Can you work these out from the model? Positions are in its coordinate system, mm. Face numbers are marked on the shaded views. A direction names the side the tool comes from. Coordinates: 2 decimals unless noted, no trailing zeros. Write each loop counter-clockwise with the first axis right and the second up, starting at its lowest first coordinate (ties: lowest second). Pieces come first, ordered by that corner, then holes. Notation, with made-up numbers: M 84.25,28 L 125.25,28 A17 ccw 125.25,46 Z; hole C -39,-28 d11. An arc over 180 degrees is marked long. Use one line per item in the form item = value. Start each with the question number.
```python
from build123d import *

# Parameters (mm, degrees)
SKETCH_1_W          = 32.677388302
SKETCH_1_H          = 8
EXTRUDE_1_DEPTH     = 3
SKETCH_2_R          = 1.5
CUT_EXTRUDE_1_DEPTH = 4
SKETCH_3_R          = 6
EXTRUDE_2_DEPTH     = 8
SKETCH_4_R          = 4
CUT_EXTRUDE_2_DEPTH = 9
EXTRUDE_3_DEPTH     = 8
SKETCH_6_W          = 6
SKETCH_6_H          = 6
EXTRUDE_4_DEPTH     = 8
SKETCH_8_W          = 3
SKETCH_8_H          = 10.466633743
CUT_EXTRUDE_5_DEPTH = 9
SKETCH_9_R          = 1.5
CUT_EXTRUDE_6_DEPTH = 20.338694151
FILLET_1_R          = 2
FILLET_2_R          = 2


with BuildPart() as part:
    # Sketch 1 → Extrude 1 (new body)
    with BuildSketch(Plane.XY):
        with Locations((-3.726697353, 26.358574689)):
            Rectangle(SKETCH_1_W, SKETCH_1_H)
    extrude(amount=-EXTRUDE_1_DEPTH)

    # Sketch 2 → Cut-Extrude 1 (cut, through all)
    with BuildSketch(Plane.XY):
        with Locations((-12.726697353, 26.358574689)):
            Circle(SKETCH_2_R)
        with Locations((5.273302647, 26.358574689)):
            Circle(SKETCH_2_R)
    extrude(amount=-CUT_EXTRUDE_1_DEPTH, mode=Mode.SUBTRACT)



with BuildPart() as body_2:
    # Sketch 3 → Extrude 2 (new body)
    with BuildSketch(Plane.XZ.offset(-22.358574689)):
        with Locations((-3.726697353, 6)):
            Circle(SKETCH_3_R)
    extrude(amount=-EXTRUDE_2_DEPTH)

    # Sketch 4 → Cut-Extrude 2 (cut, through all)
    with BuildSketch(Plane.XZ.offset(-22.358574689)):
        with Locations((-3.726697353, 6)):
            Circle(SKETCH_4_R)
    extrude(amount=-CUT_EXTRUDE_2_DEPTH, mode=Mode.SUBTRACT)


with BuildPart() as part_1:
    add(part.part)

    add(body_2.part)  # Extrude 3 merges body 2
    # Sketch 5 → Extrude 3 (add)
    with BuildSketch(Plane.XZ.offset(-22.358574689)):
        Polygon((-3.726697353, 0), (-9.726697353, 6), (-9.726697353, 0), align=None)
        Polygon((2.273302647, 6), (-3.726697353, 0), (2.273302647, 0), align=None)
    extrude(amount=-EXTRUDE_3_DEPTH)

    # Sketch 6 → Extrude 4 (add)
    with BuildSketch(Plane.XZ.offset(-22.358574689)):
        with Locations((-3.726697353, 13)):
            Rectangle(SKETCH_6_W, SKETCH_6_H)
    extrude(amount=-EXTRUDE_4_DEPTH)

    # Sketch 8 → Cut-Extrude 5 (cut, through all)
    with BuildSketch(Plane.XZ.offset(-22.358574689)):
        with Locations((-3.726697353, 11.233316872)):
            Rectangle(SKETCH_8_W, SKETCH_8_H)
    extrude(amount=-CUT_EXTRUDE_5_DEPTH, mode=Mode.SUBTRACT)

    # Sketch 9 → Cut-Extrude 6 (cut, through all)
    with BuildSketch(Plane(origin=(-0.726697353, 0, 0), x_dir=(0, 0, -1), z_dir=(1, 0, 0))):
        with Locations((-13.598076211, 26.358574689)):
            Circle(SKETCH_9_R)
    extrude(amount=-CUT_EXTRUDE_6_DEPTH, mode=Mode.SUBTRACT)

    # Fillet 1
    fillet_1_edges = [part_1.edges().sort_by_distance(p)[0] for p in [
        (12.611996798, 22.358574689, -1.5),
        (-20.065391504, 22.358574689, -1.5),
        (-20.065391504, 30.358574689, -1.5),
        (12.611996798, 30.358574689, -1.5),
    ]]
    fillet(fillet_1_edges, radius=FILLET_1_R)

    # Fillet 2
    fillet_2_edges = [part_1.edges().sort_by_distance(p)[0] for p in [
        (-1.476697353, 22.358574689, 16),
        (-1.476697353, 30.358574689, 16),
        (-5.976697353, 30.358574689, 16),
        (-5.976697353, 22.358574689, 16),
    ]]
    fillet(fillet_2_edges, radius=FILLET_2_R)


solid = part_1.part
```
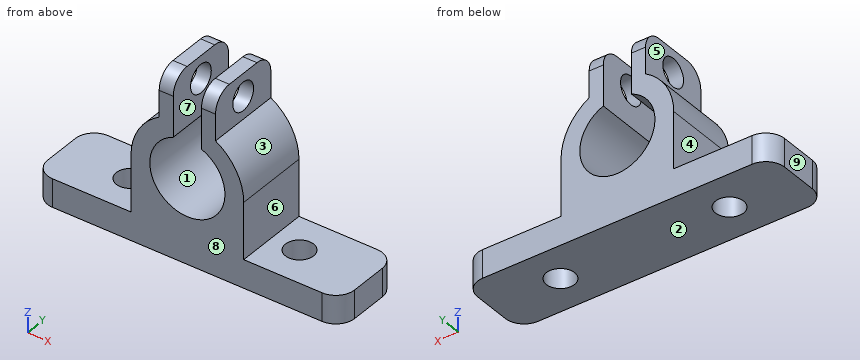
1) Suppose I cut it at A-A on x = -6. Please give me the cut outline in (y, z).
2) Suppose I cut it at D-D on z = 13. Please give me the cut outline in (x, y).
3) Suppose I cut it at C-C on z = 3.75. Please give me the cut outline in (x, y), and give its area (3 significant figures).
4) If we mould it in two halves opening along X, with no side actions, what happens to the marked faces 1, 2, 3 and 4? For each: +X half, -X half, draft (parallel to the pull), parting line (faces both ways), or undercut.
5) Will these pins go through, and if not, where does the flat tip stop? pin 1 Ø3 at (y, z) = (28, 11.5) entering from +X; pin 2 Ø4 at (x, y) = (8, 26) entering from +Z; pin 3 Ø3 at (y, z) = (27.5, 4) entering from -X.
6) Suppose I cut it at B-B on y = 25.25. State how many separate pieces and enclosed holes the cut face has, and give its area (3 significant figures).
7) Please list where these lines run through material, in increasing order: line 1 (X direction, y = 25, z = 15.25); line 2 (Z direction, x = -6.5, y = 26.5); line 3 (X direction, y = 29.5, z = 6.25).
8) Which directions (+Z, -Z, +X, -X, +Y, -Y) give clear straight access to the entire face, cutting with the end or side of a thin tool? Please do the marked faces 5, 6, 7, 8 and 9.
Computed values:
q1.outline = M 22.36,-3 L 30.36,-3 L 30.36,2.71 L 22.36,2.71 Z; M 22.36,9.29 L 30.36,9.29 L 30.36,14 A2 ccw 28.36,16 L 24.36,16 A2 ccw 22.36,14 Z; hole C 26.36,13.6 d3
q2.outline = M -6.73,22.36 L -5.23,22.36 L -5.23,24.98 L -6.73,24.98 Z; M -6.73,27.73 L -5.23,27.73 L -5.23,30.36 L -6.73,30.36 Z; M -2.23,22.36 L -0.73,22.36 L -0.73,24.98 L -2.23,24.98 Z; M -2.23,27.73 L -0.73,27.73 L -0.73,30.36 L -2.23,30.36 Z
q3.outline = M -9.73,22.36 L -7.03,22.36 L -7.03,30.36 L -9.73,30.36 Z; M -0.42,22.36 L 2.27,22.36 L 2.27,30.36 L -0.42,30.36 Z
q3.area = 43.1 mm²
q4.face_1 = undercut
q4.face_2 = draft
q4.face_3 = +X half
q4.face_4 = -X half
q5.pin_1 = 0.75
q5.pin_2 = 0
q5.pin_3 = -9.73
q6.separate_pieces = 5
q6.enclosed_holes = 0
q6.area = 165 mm²
q7.line_1 = -6.73 to -5.23, -2.23 to -0.73
q7.line_2 = -3 to 3.12, 8.88 to 12.1, 15.09 to 16
q7.line_3 = -9.72 to -7.72, 0.27 to 2.27
q8.face_5 = +Z, -X, +Y, -Y
q8.face_6 = +Z, +X, +Y, -Y
q8.face_7 = +Z, +Y, -Y
q8.face_8 = +Z, -Z, +X, -X, -Y
q8.face_9 = +Z, -Z, -X, +Y, -Y
